```python
from build123d import *

# Parameters (mm, degrees)
SKETCH_1_R      = 56
SKETCH_1_R_2    = 47.5
SKETCH_1_R_3    = 1.55
EXTRUDE_1_DEPTH = 7


with BuildPart() as part:
    # 草图1 → 凸台-拉伸1 (new body)
    with BuildSketch(Plane.XY):
        Circle(SKETCH_1_R)
        Circle(SKETCH_1_R_2, mode=Mode.SUBTRACT)
        with Locations((0, 52)):
            Circle(SKETCH_1_R_3, mode=Mode.SUBTRACT)
        with Locations((11.571088566, 50.696251433)):
            Circle(SKETCH_1_R_3, mode=Mode.SUBTRACT)
        with Locations((22.561954434, 46.850381131)):
            Circle(SKETCH_1_R_3, mode=Mode.SUBTRACT)
        with Locations((32.421469697, 40.655237088)):
            Circle(SKETCH_1_R_3, mode=Mode.SUBTRACT)
        with Locations((40.655237088, 32.421469697)):
            Circle(SKETCH_1_R_3, mode=Mode.SUBTRACT)
        with Locations((46.850381131, 22.561954434)):
            Circle(SKETCH_1_R_3, mode=Mode.SUBTRACT)
        with Locations((50.696251433, 11.571088566)):
            Circle(SKETCH_1_R_3, mode=Mode.SUBTRACT)
        with Locations((52, 0)):
            Circle(SKETCH_1_R_3, mode=Mode.SUBTRACT)
        with Locations((50.696251433, -11.571088566)):
            Circle(SKETCH_1_R_3, mode=Mode.SUBTRACT)
        with Locations((46.850381131, -22.561954434)):
            Circle(SKETCH_1_R_3, mode=Mode.SUBTRACT)
        with Locations((40.655237088, -32.421469697)):
            Circle(SKETCH_1_R_3, mode=Mode.SUBTRACT)
        with Locations((32.421469697, -40.655237088)):
            Circle(SKETCH_1_R_3, mode=Mode.SUBTRACT)
        with Locations((22.561954434, -46.850381131)):
            Circle(SKETCH_1_R_3, mode=Mode.SUBTRACT)
        with Locations((11.571088566, -50.696251433)):
            Circle(SKETCH_1_R_3, mode=Mode.SUBTRACT)
        with Locations((0, -52)):
            Circle(SKETCH_1_R_3, mode=Mode.SUBTRACT)
        with Locations((-11.571088566, -50.696251433)):
            Circle(SKETCH_1_R_3, mode=Mode.SUBTRACT)
        with Locations((-22.561954434, -46.850381131)):
            Circle(SKETCH_1_R_3, mode=Mode.SUBTRACT)
        with Locations((-32.421469697, -40.655237088)):
            Circle(SKETCH_1_R_3, mode=Mode.SUBTRACT)
        with Locations((-40.655237088, -32.421469697)):
            Circle(SKETCH_1_R_3, mode=Mode.SUBTRACT)
        with Locations((-46.850381131, -22.561954434)):
            Circle(SKETCH_1_R_3, mode=Mode.SUBTRACT)
        with Locations((-50.696251433, -11.571088566)):
            Circle(SKETCH_1_R_3, mode=Mode.SUBTRACT)
        with Locations((-52, 0)):
            Circle(SKETCH_1_R_3, mode=Mode.SUBTRACT)
        with Locations((-50.696251433, 11.571088566)):
            Circle(SKETCH_1_R_3, mode=Mode.SUBTRACT)
        with Locations((-46.850381131, 22.561954434)):
            Circle(SKETCH_1_R_3, mode=Mode.SUBTRACT)
        with Locations((-40.655237088, 32.421469697)):
            Circle(SKETCH_1_R_3, mode=Mode.SUBTRACT)
        with Locations((-32.421469697, 40.655237088)):
            Circle(SKETCH_1_R_3, mode=Mode.SUBTRACT)
        with Locations((-22.561954434, 46.850381131)):
            Circle(SKETCH_1_R_3, mode=Mode.SUBTRACT)
        with Locations((-11.571088566, 50.696251433)):
            Circle(SKETCH_1_R_3, mode=Mode.SUBTRACT)
    extrude(amount=EXTRUDE_1_DEPTH)


solid = part.part
```
Work out the finished part from the listing and answer in its coordinate system (mm). Give positions to 0.01 mm unless a question says otherwise; leave off trailing zeros. Loops run counter-clockwise (first coordinate to the right, second up) from the corner with the lowest first, then second, coordinate; pieces in that order, holes last. Notation, with made-up numbers: (51.5, 41.25) - (69.5, 41.25) arc R31 ccw to (69.5, 79.25) - close; hole circle Ø1 at (-10.5, -2). An arc over 180 degrees is marked (long way). Use CSV: the item, a comma, the result in double quotes. Start each with the question number.
(1) Find section D-D, the plane z = 2. Count the separate pieces of the cut face and the enclosed holes in it, plus the area to 3 significant figures.
(2) Find section C-C, the plane x = -7.5. Determine the outline of the cut face in (y, z), plus the area to 3 significant figures.
(3) Determine the mould class of faces 1 (the face through (47.68, 23.87, 3.45)), 2 (the face through (51.73, -21.45, 3.45)), 3 (the face through (-10.3, -46.37, 3.45)), 4 (the face through (-29, 38, 7)) for opening direction X: released by +X, released by -X, zero draft, split by the parting line, or undercut.
(4) Find section B-B, the plane y = 0. Determine the outline of the cut face in (x, z), plus the area to 3 significant figures.
(5) Find the intervals of material crossed by L1, parallel to Y at x = 0, z = 3; L2, parallel to X at y = -33.5, z = 4; L3, parallel to X at y = 1, z = 2.5, in increasing order.
(6) Each of these flat-tipped pins is pushed along its axis until it touches: pin 1 (2 mm diameter, centred on x = 11.5, z = 3, fed in from -Y); pin 2 (1 mm diameter, centred on x = -19, z = 5.5, fed in from -Y); pin 3 (2 mm diameter, centred on y = 33, z = 1, fed in from -X). Where does it stop, or does it pass through?
(7) Find section A-A, the plane x = -32.5. Determine the outline of the cut face in (y, z).
Results found:
1,separate pieces,"1"
1,enclosed holes,"29"
1,area,"2,550 mm^2"
2,outline,"(-55.5, 0) - (-46.9, 0) - (-46.9, 7) - (-55.5, 7) - close; (46.9, 0) - (55.5, 0) - (55.5, 7) - (46.9, 7) - close"
2,area,"120 mm^2"
3,face 1,"undercut"
3,face 2,"split by the parting line"
3,face 3,"undercut"
3,face 4,"zero draft"
4,outline,"(-56, 0) - (-53.55, 0) - (-53.55, 7) - (-56, 7) - close; (-50.45, 0) - (-47.5, 0) - (-47.5, 7) - (-50.45, 7) - close; (47.5, 0) - (50.45, 0) - (50.45, 7) - (47.5, 7) - close; (53.55, 0) - (56, 0) - (56, 7) - (53.55, 7) - close"
4,area,"75.6 mm^2"
5,L1,"-56 to -53.55, -50.45 to -47.5, 47.5 to 50.45, 53.55 to 56"
5,L2,"-44.87 to -41.77, -39.54 to -33.67, 33.67 to 39.54, 41.77 to 44.87"
5,L3,"-55.99 to -53.18, -50.82 to -47.49, 47.49 to 50.82, 53.18 to 55.99"
6,pin 1,"y = -55.01"
6,pin 2,"y = -52.86"
6,pin 3,"x = -45.96"
7,outline,"(-45.6, 0) - (-42.2, 0) - (-42.2, 7) - (-45.6, 7) - close; (-39.11, 0) - (-34.64, 0) - (-34.64, 7) - (-39.11, 7) - close; (34.64, 0) - (39.11, 0) - (39.11, 7) - (34.64, 7) - close; (42.2, 0) - (45.6, 0) - (45.6, 7) - (42.2, 7) - close"
